from build123d import *

# Parameters (mm, degrees)
F0_W      = 914.4
F0_H      = 609.6
F1_DEPTH  = 609.6
F3_DEPTH  = 914.401
F4_R      = 127
F5_DEPTH  = 381
F6_W      = 203.2
F6_H      = 203.2
F7_DEPTH  = 38.1
F8_R      = 12.7
F10_DEPTH = 19.05
F11_W     = 76.2
F11_H     = 95.25
F12_DEPTH = 6.35


with BuildPart() as f1:
    # F0 (on Top) → F1 (new body)
    with BuildSketch(Plane.XY):
        with Locations((457.2, 304.8)):
            Rectangle(F0_W, F0_H)
    extrude(amount=F1_DEPTH)

    # F2 (on face) → F3 (cut, through all)
    with BuildSketch(Plane(origin=(0, 0, 0), x_dir=(0, -1, 0), z_dir=(-1, 0, 0))):
        Polygon((0, 609.6), (-304.8, 609.6), (0, 0), align=None)
    extrude(amount=-F3_DEPTH, mode=Mode.SUBTRACT)

    # F4 (on face) → F5 (cut)
    with BuildSketch(Plane(origin=(0, 0, 0), x_dir=(1, 0, 0), z_dir=(0, -0.894427191, 0.4472135955))):
        with Locations((228.6, 340.776759771)):
            Circle(F4_R)
        with Locations((685.8, 340.776759771)):
            Circle(F4_R)
    extrude(amount=-F5_DEPTH, mode=Mode.SUBTRACT)

    # F6 (on face) → F7 (join)
    with BuildSketch(Plane(origin=(0, 609.6, 0), x_dir=(-1, 0, 0), z_dir=(0, 1, 0))):
        with Locations((-228.6, 203.2)):
            Rectangle(F6_W, F6_H)
    extrude(amount=F7_DEPTH)

    # F8
    f8_edges = [f1.edges().sort_by_distance(p)[0] for p in [
        (127, 647.7, 203.2),
        (228.6, 647.7, 304.8),
        (330.2, 647.7, 203.2),
        (228.6, 647.7, 101.6),
    ]]
    fillet(f8_edges, radius=F8_R)

    # F9 (on face) → F10 (join)
    with BuildSketch(Plane(origin=(0, 609.6, 0), x_dir=(-1, 0, 0), z_dir=(0, 1, 0))):
        Polygon((0, 609.6), (-914.4, 609.6), (-914.4, 0), (-229.87, 0), (-229.87, 95.25), (-336.55, 95.25), (-336.55, 311.15), (-120.65, 311.15), (-120.65, 95.25), (-153.67, 95.25), (-153.67, 0), (0, 0), align=None)
    extrude(amount=F10_DEPTH)

    # F11 (on face) → F12 (join)
    with BuildSketch(Plane(origin=(0, 628.65, 0), x_dir=(-1, 0, 0), z_dir=(0, 1, 0))):
        with Locations((-191.77, 47.625)):
            Rectangle(F11_W, F11_H)
    extrude(amount=-F12_DEPTH)


solid = f1.part
Could you check a few things on this model? Use its own coordinates, in mm. A direction names the side the tool comes from. Round coordinates to 2 decimals unless told otherwise and drop trailing zeros. Order: outer loops, then holes, each group sorted by start corner. A loop starts at its lowest first (then second) coordinate and runs counter-clockwise, first axis right, second up.
Q1. Thinking about a two-plate mould opening in Y: for faces 1 (the face through (330.2, 622, 202)), 2 (the face through (450.799, 154.534, 309.067)), 3 (the face through (287.2, 270.02, 120.02)), which applies, released by +Y, released by -Y, zero draft, split by the parting line, or undercut?
Geometry says:
face 1: zero draft
face 2: released by -Y
face 3: undercut
Q2. Please list where these lines run through material, in increasing order: probe 1 along X at (y, z) = (401, 283); probe 2 along X at (y, z) = (315.5, 336.5); probe 3 along Z at (x, y) = (775, 289.5).
Geometry says:
probe 1: x = 0 to 140.71, 316.49 to 597.91, 773.69 to 914.4
probe 2: x = 0 to 151.99, 305.21 to 609.19, 762.41 to 914.4
probe 3: z = 0 to 135.18, 337.32 to 579
Q3. I'm going to push flat-ended pins straight in: P1, Ø6, axis at x = 209.5, z = 216, coming from the -Y side; P2, Ø1.5, axis at x = 346.5, z = 225, coming from the +Y side; P3, Ø5.5, axis at x = 200, y = 619, coming from the -Z side. Where does each tip first touch, or does it pass through?
Geometry says:
P1: stops at y = 532.47
P2: stops at y = 628.65
P3: stops at z = 101.6
Q4. Which directions (+Z, -Z, +X, -X, +Y, -Y) give clear straight access to the entire face, cutting with the end or side of a thin tool? Please do faces 4 (the face through (914.4, 380, 309)), 5 (the face through (127, 622, 202)), 6 (the face through (0, 380, 301)), 7 (the face through (684.02, 493.97, 136)), 8 (the face through (192, 622.3, 48)).
Geometry says:
face 4: +Z, -Z, +X, +Y, -Y
face 5: +Y
face 6: +Z, -Z, -X, +Y, -Y
face 7: none
face 8: -Z
Q5. Imagine slicing it at A-A, the plane x = 583. List the corners of the cut face in (y, z) for me, then the cut area to 3 significant figures.
Geometry says:
outline: (0, 0) - (628.65, 0) - (628.65, 609.6) - (304.8, 609.6) - (185.75, 371.5) - (526.53, 201.11) - (459.83, 67.71) - (119.05, 238.1) - close
area: 233,000 mm2
Q6. Imagine slicing it at C-C, the plane y = 61.5. List the corners of the cut face in (x, z) for me, then the cut area to 3 significant figures.
Geometry says:
outline: (0, 0) - (914.4, 0) - (914.4, 123) - (0, 123) - close
area: 112,000 mm2
Q7. Imagine slicing it at B-B, the plane z = 554. List the corners of the cut face in (x, y) for me.
Geometry says:
outline: (0, 277) - (914.4, 277) - (914.4, 628.65) - (0, 628.65) - close
Q8. Imagine slicing it at D-D, the plane y = 388. State how many separate pieces and enclosed holes the cut face has, then the cut area to 3 significant figures.
Geometry says:
separate pieces: 1
enclosed holes: 2
area: 444,000 mm2
